Could you check a few things on this model? Use its own coordinates, in mm. Face numbers are marked on the shaded views. A direction names the side the tool comes from. Give positions to 0.01 mm unless a question says otherwise; leave off trailing zeros. Write each loop counter-clockwise with the first axis right and the second up, starting at its lowest first coordinate (ties: lowest second). Pieces come first, ordered by that corner, then holes. Notation, with made-up numbers: (88, 24.25) - (131, 24.25) arc R22 ccw to (131, 55.25) - close; hole circle Ø9 at (-26.75, 32.5). An arc over 180 degrees is marked (long way). Answer as a JSON object with one key per item and string values. Group by question number.
```python
from build123d import *

# Parameters (mm, degrees)
F0_R      = 21.4164389033
F1_DEPTH  = 127
F2_W      = 42.8202235004
F2_H      = 103.2743248374
F3_DEPTH  = 17.78
F5_DEPTH  = 17.78
F6_R      = 7.3683109371
F7_DEPTH  = 273
F8_R      = 10.2975296605
F9_DEPTH  = 127.001
F11_DEPTH = 17.78
F13_DEPTH = 17.78
F14_R     = 10.2092328794
F15_DEPTH = 127.001


# Not quite as in the source:
# - an extrude ends at something that could not be found from the text; its depth is read off the source's solid


with BuildPart() as f1:
    # F0 (on Front) → F1 (new body)
    with BuildSketch(Plane.XZ):
        with Locations((25.1603480428, 31.716234982)):
            Circle(F0_R)
    extrude(amount=F1_DEPTH)

    # F2 (on face) → F3 (join)
    with BuildSketch(Plane(origin=(0, 0, 0), x_dir=(-1, 0, 0), z_dir=(0, 1, 0))):
        with Locations((-25.1603480428, 83.8739453241)):
            Rectangle(F2_W, F2_H)
    extrude(amount=-F3_DEPTH)

    # F4 (on face) → F5 (join)
    with BuildSketch(Plane.XZ.offset(127)):
        Polygon((3.7453082572, 31.961033423), (46.5753878285, 31.961033423), (46.636801213, 135.9289437532), (3.7453082572, 135.9289437532), align=None)
    extrude(amount=-F5_DEPTH)

    # F6 (on Front) → F7 (cut, through all)
    with BuildSketch(Plane.XZ):
        with Locations((25.2368301153, 31.4926542342)):
            Circle(F6_R)
    extrude(amount=-F7_DEPTH, mode=Mode.SUBTRACT)

    # F8 (on Front) → F9 (cut, through all)
    with BuildSketch(Plane.XZ):
        with Locations((24.5855599642, 32.795201987)):
            Circle(F8_R)
    extrude(amount=F9_DEPTH, mode=Mode.SUBTRACT)

    # F10 (on face) → F11 (join)
    with BuildSketch(Plane.XZ.offset(127)):
        with BuildLine():
            Line((3.7453082572, 135.9289437532), (46.636801213, 135.9289437532))
            ThreePointArc((46.636801213, 135.9289437532), (25.1910547351, 157.3873618801), (3.7453082572, 135.9289437532))
        make_face()
    extrude(amount=-F11_DEPTH)

    # F12 (on face) → F13 (join)
    with BuildSketch(Plane(origin=(0, 0, 0), x_dir=(-1, 0, 0), z_dir=(0, 1, 0))):
        with BuildLine():
            Line((-46.5704597931, 135.5111077428), (-3.7502362926, 135.5111077428))
            ThreePointArc((-3.7502362926, 135.5111077428), (-25.1603480428, 156.921219493), (-46.5704597931, 135.5111077428))
        make_face()
    extrude(amount=-F13_DEPTH)

    # F14 (on face) → F15 (cut, through all)
    with BuildSketch(Plane.XZ.offset(127)):
        with Locations((25.1910547351, 135.9416116608)):
            Circle(F14_R)
    extrude(amount=-F15_DEPTH, mode=Mode.SUBTRACT)


solid = f1.part
```
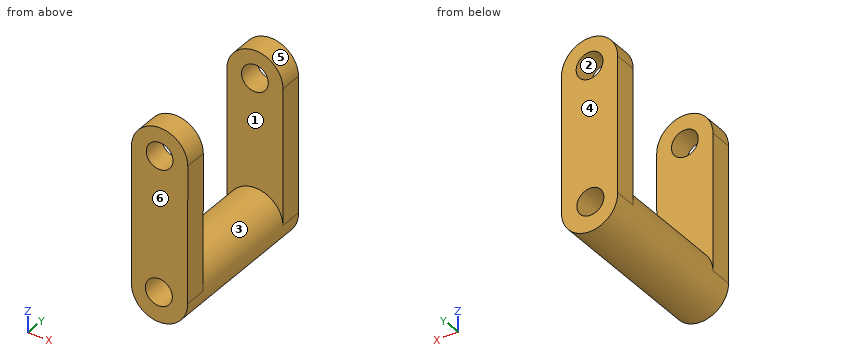
(1) If we mould it in two halves opening along Y, with no side actions, what happens to the marked faces 1, 2, 3 and 4? For each: +Y half, -Y half, draft (parallel to the pull), parting line (faces both ways), or undercut.
(2) For the marked faces 5 and 6, which set-ups out of +Z, -Z, +X, -X, +Y, -Y let a thin tool reach every point of the face, with its end or its side?
(3) I want a section at D-D, the plane x = 37.5. Please give me the cut outline in (y, z).
(4) I want a section at C-C, the plane z = 97. Please give me the cut outline in (x, y), and give its area (3 significant figures).
(5) I want a section at B-B, the plane x = 25. Please give me the cut outline in (y, z), and give its area (3 significant figures).
(6) I want a section at A-A, the plane z = 141.5. Please give me the cut outline in (x, y).
(7) Will these pins go through, and if not, where does the flat tip stop? P1, Ø5.5, axis at y = -11.5, z = 106, coming from the -X side; P2, Ø1, axis at x = 28.5, z = 65.5, coming from the +Y side; P3, Ø6, axis at x = 31, z = 139, coming from the -Y side; P4, Ø5.5, axis at y = -12.5, z = 77, coming from the +X side.
(8) I need wall thicknesses on L1, parallel to Y at x = 36, z = 97; L2, parallel to Z at x = 22, y = -85; L3, parallel to X at y = -114.5, z = 87. Which ranges of each line are inside material? Lowest first, please.
Entries:
{
 "1": {"face 1": "undercut", "face 2": "draft", "face 3": "undercut", "face 4": "+Y half"},
 "2": {"face 5": "+Z, +Y", "face 6": "+Z, -Z, +X, -X, -Y"},
 "3": {"outline": "(-127, 14.21) - (0, 14.21) - (0, 153.01) - (-17.78, 153.01) - (-17.78, 49.22) - (-109.22, 49.22) - (-109.22, 153.5) - (-127, 153.5) - close"},
 "4": {"outline": "(3.75, -127) - (46.61, -127) - (46.61, -109.22) - (3.75, -109.22) - close; (3.75, -17.78) - (46.57, -17.78) - (46.57, 0) - (3.75, 0) - close", "area": "1,520 mm^2"},
 "5": {"outline": "(-127, 10.3) - (0, 10.3) - (0, 22.51) - (-127, 22.51) - close; (-127, 43.08) - (0, 43.08) - (0, 125.73) - (-17.78, 125.73) - (-17.78, 53.13) - (-109.22, 53.13) - (-109.22, 125.73) - (-127, 125.73) - close; (-127, 146.15) - (-109.22, 146.15) - (-109.22, 157.39) - (-127, 157.39) - close; (-17.78, 146.15) - (0, 146.15) - (0, 156.92) - (-17.78, 156.92) - close", "area": "5,800 mm^2"},
 "6": {"outline": "(4.48, -127) - (16.63, -127) - (16.63, -109.22) - (4.48, -109.22) - close; (4.6, -17.78) - (16.63, -17.78) - (16.63, 0) - (4.6, 0) - close; (33.75, -127) - (45.9, -127) - (45.9, -109.22) - (33.75, -109.22) - close; (33.75, -17.78) - (45.72, -17.78) - (45.72, 0) - (33.75, 0) - close"},
 "7": {"P1": "x = 3.75", "P2": "y = 0", "P3": "through", "P4": "x = 46.57"},
 "8": {"L1": "-127 to -109.22, -17.78 to 0", "L2": "10.53 to 22.83, 42.76 to 52.9", "L3": "3.75 to 46.61"}
}
